```python
from build123d import *

# Parameters (mm, degrees)
SKETCH1_R           = 2.413
SKETCH1_R_2         = 0.75
BOSS_EXTRUDE1_DEPTH = 1.5
SKETCH2_R           = 3.2
SKETCH2_R_2         = 2.413
BOSS_EXTRUDE2_DEPTH = 4
FILLET1_R           = 1


with BuildPart() as part:
    # Sketch1 → Boss-Extrude1 (new body)
    with BuildSketch(Plane(origin=(0, 0, 0), x_dir=(1, 0, 0), z_dir=(0, 1, 0))):
        Polygon((-1.5, 19), (-3.5, 3.5), (-19, 1.5), (-19, -1.5), (-3.5, -3.5), (-1.5, -19), (1.5, -19), (3.5, -3.5), (19, -1.5), (19, 1.5), (3.5, 3.5), (1.5, 19), align=None)
        Circle(SKETCH1_R, mode=Mode.SUBTRACT)
        with Locations((8, 0)):
            Circle(SKETCH1_R_2, mode=Mode.SUBTRACT)
        with Locations((11, 0)):
            Circle(SKETCH1_R_2, mode=Mode.SUBTRACT)
        with Locations((14, 0)):
            Circle(SKETCH1_R_2, mode=Mode.SUBTRACT)
        with Locations((17, 0)):
            Circle(SKETCH1_R_2, mode=Mode.SUBTRACT)
        with Locations((0, -8)):
            Circle(SKETCH1_R_2, mode=Mode.SUBTRACT)
        with Locations((0, -11)):
            Circle(SKETCH1_R_2, mode=Mode.SUBTRACT)
        with Locations((0, -14)):
            Circle(SKETCH1_R_2, mode=Mode.SUBTRACT)
        with Locations((0, -17)):
            Circle(SKETCH1_R_2, mode=Mode.SUBTRACT)
        with Locations((-8, 0)):
            Circle(SKETCH1_R_2, mode=Mode.SUBTRACT)
        with Locations((-11, 0)):
            Circle(SKETCH1_R_2, mode=Mode.SUBTRACT)
        with Locations((-14, 0)):
            Circle(SKETCH1_R_2, mode=Mode.SUBTRACT)
        with Locations((-17, 0)):
            Circle(SKETCH1_R_2, mode=Mode.SUBTRACT)
        with Locations((0, 8)):
            Circle(SKETCH1_R_2, mode=Mode.SUBTRACT)
        with Locations((0, 11)):
            Circle(SKETCH1_R_2, mode=Mode.SUBTRACT)
        with Locations((0, 14)):
            Circle(SKETCH1_R_2, mode=Mode.SUBTRACT)
        with Locations((0, 17)):
            Circle(SKETCH1_R_2, mode=Mode.SUBTRACT)
    extrude(amount=BOSS_EXTRUDE1_DEPTH)

    # Sketch2 → Boss-Extrude2 (add)
    with BuildSketch(Plane.XZ):
        Circle(SKETCH2_R)
        Circle(SKETCH2_R_2, mode=Mode.SUBTRACT)
    extrude(amount=BOSS_EXTRUDE2_DEPTH)

    # Fillet1
    fillet1_edges = [part.edges().sort_by_distance(p)[0] for p in [
        (-1.5, 0.75, 19),
        (-3.5, 0.75, 3.5),
        (-19, 0.75, 1.5),
        (-19, 0.75, -1.5),
        (-3.5, 0.75, -3.5),
        (-1.5, 0.75, -19),
        (1.5, 0.75, -19),
        (3.5, 0.75, -3.5),
        (19, 0.75, -1.5),
        (19, 0.75, 1.5),
        (3.5, 0.75, 3.5),
        (1.5, 0.75, 19),
    ]]
    fillet(fillet1_edges, radius=FILLET1_R)


solid = part.part
```
For this review, take the finished solid that the model builds, in its own axes (mm). A direction names the side the tool comes from. Coordinates: 2 decimals unless noted, no trailing zeros. Order: outer loops, then holes, each group sorted by start corner. A loop starts at its lowest first (then second) coordinate and runs counter-clockwise, first axis right, second up. Notation, with made-up numbers: (65.5, -23.5) - (76.5, -23.5) arc R12 ccw to (76.5, -18.5) - close; hole circle Ø10 at (-33.75, 67). An arc over 180 degrees is marked (long way). Answer as a JSON object with one key per item and string values. Group by question number.
1. The part is to be moulded in two halves that separate along Z. For faces 3 (the flat face through (-2.494, 0.74, -11.294)), 4 (the cylindrical face through (-8.75, 0.74, -0.03)), 5 (the cylindrical face through (1.289, 0.76, 18.744)), say which applies: pulls with the +Z half, pulls with the -Z half, needs draft (parallel to the pull), parting line crosses it, or undercut.
2. We need section A-A on z = 17. State the section outline as (x, y) points.
3. Clearance check with flat-ended pins moving along their axes: P1, Ø0.9, axis at x = 14, z = 0, coming from the -Y side; P2, Ø2.5, axis at x = 0, z = 8, coming from the -Y side; P3, Ø2, axis at x = 6.5, y = 1, coming from the -Z side. State where each tip first meets the part, or that it passes through.
4. We need section B-B on x = 17. State the section outline as (y, z) points.
5. We need section D-D on y = 0.95. Give the number of separate pieces and of enclosed holes in the cut face, then the cut area to 3 significant figures.
6. We need section C-C on y = -1.55. State the section outline as (x, z) points.
7. For probe 1 along Y at (x, z) = (-7, 2); probe 2 along Z at (x, y) = (-17, 1.05); probe 3 along Z at (x, y) = (-8, 0.65), list the stretches that pass through material, from the lowest coordinate up.
8. For faces 1 (the flat face through (3, 0, 3)), 2 (the cylindrical face through (-0.163, 0.74, 8.732)), list the 3-axis set-ups (+Z, -Z, +X, -X, +Y, -Y) from which the entire face can be reached by the end or side of a thin tool; tool diameter is ignored.
Final values:
{
 "1": {"face 3": "pulls with the -Z half", "face 4": "undercut", "face 5": "pulls with the +Z half"},
 "2": {"outline": "(-1.76, 0) - (-0.75, 0) - (-0.75, 1.5) - (-1.76, 1.5) - close; (0.75, 0) - (1.76, 0) - (1.76, 1.5) - (0.75, 1.5) - close"},
 "3": {"P1": "through", "P2": "y = 0", "P3": "z = -3.24"},
 "4": {"outline": "(0, -1.76) - (1.5, -1.76) - (1.5, -0.75) - (0, -0.75) - close; (0, 0.75) - (1.5, 0.75) - (1.5, 1.76) - (0, 1.76) - close"},
 "5": {"separate pieces": "1", "enclosed holes": "17", "area": "312 mm²"},
 "6": {"outline": "circle Ø6.4 at (0, 0); hole circle Ø4.83 at (0, 0)"},
 "7": {"probe 1": "0 to 1.5", "probe 2": "-1.76 to -0.75, 0.75 to 1.76", "probe 3": "-2.92 to -0.75, 0.75 to 2.92"},
 "8": {"face 1": "-Y", "face 2": "+Y, -Y"}
}
